Input: part model. Units: mm. Frame: model coordinates. A direction names the side the tool comes from. Coordinates: 2 decimals unless noted, no trailing zeros. Loops run counter-clockwise (first coordinate to the right, second up) from the corner with the lowest first, then second, coordinate; pieces in that order, holes last. Notation, with made-up numbers: (-35.5, -12) - (23.5, -12) arc R25 cw to (23.5, 15) - close; hole circle Ø4 at (-32, 5.25). An arc over 180 degrees is marked (long way). Use a Markdown table: item, result. Add a question column.
1. Access query for faces 1 (the face through (123.825, 47, 3)), 2 (the face through (93.967, 92, 3)), 3 (the face through (-82, 74.261, 3)). Directions: +Z, -Z, +X, -X, +Y, -Y. A direction counts if a zero-diameter tool reaches every point of the face in a straight line with its end or side. Return the directions, or none.
2. Ray query, L1, parallel to Y at x = 113, z = 2.5; L2, parallel to X at y = 88.5, z = 4.25; L3, parallel to X at y = 78, z = 5 (3 decimals). Return the intervals inside material, ascending. Write a range as [from, to].
3. Section query A-A on y = 14. Return the cut outline in (x, z).
4. Draft query along X for faces 4 (the face through (127, 38, 3)), 5 (the face through (62.23, 92, 3)), 6 (the face through (-19, 0, 3)). Return one class per face: released by +X, released by -X, zero draft, split by the parting line, or undercut.
5. Contact query for flat-ended pins moving along their axis: P1, Ø1.5, axis at y = 42.5, z = 4, coming from the -X side; P2, Ø3, axis at y = 25, z = 3.5, coming from the +X side (3 decimals); P3, Ø0.8, axis at x = 94.5, z = 2.5, coming from the -Y side. Output: stop coordinate, or through.
```python
from build123d import *

# Parameters (mm, degrees)
BOSS_EXTRUDE1_DEPTH     = 6.35
CUT_EXTRUDE4_DEPTH      = 127
CUT_EXTRUDE4_DEPTH_BACK = 127
CUT_EXTRUDE5_DEPTH      = 127
CUT_EXTRUDE5_DEPTH_BACK = 127
SKETCH5_W               = 229.808362084
SKETCH5_H               = 77.917038349
CUT_EXTRUDE7_DEPTH      = 127
CUT_EXTRUDE7_DEPTH_BACK = 127


with BuildPart() as part:
    # Sketch1 → Boss-Extrude1 (new body)
    with BuildSketch(Plane.XY):
        Polygon((0, 0), (127, 0), (127, 101.6), (0, 101.6), (-70.692427737, 172.292427737), (-91.896861793, 151.087993682), (-91.896861793, 0), align=None)
    extrude(amount=BOSS_EXTRUDE1_DEPTH)

    # Sketch3 → Cut-Extrude4 (cut, two sides)
    with BuildSketch(Plane(origin=(0, 0, 0), x_dir=(-1, 0, 0), z_dir=(0, 0, -1))) as cut_extrude4_sk:
        Polygon((-88.9, 101.6), (-101.6, 101.6), (-101.6, 98.425), (-96.5327, 98.425), (-96.5327, 85.725), (-93.9673, 85.725), (-93.9673, 98.425), (-88.9, 98.425), align=None)
        Polygon((-57.15, 101.6), (-69.85, 101.6), (-69.85, 98.425), (-64.77, 98.425), (-64.77, 85.725), (-62.23, 85.725), (-62.23, 98.425), (-57.15, 98.425), align=None)
        Polygon((-127, 82.55), (-127, 69.85), (-123.825, 69.85), (-123.825, 74.9173), (-111.125, 74.9173), (-111.125, 77.4827), (-123.825, 77.4827), (-123.825, 82.55), align=None)
        Polygon((-127, 57.15), (-127, 44.45), (-123.825, 44.45), (-123.825, 49.5173), (-111.125, 49.5173), (-111.125, 52.0827), (-123.825, 52.0827), (-123.825, 57.15), align=None)
        Polygon((-127, 31.75), (-127, 25.4), (-127, 19.05), (-123.825, 19.05), (-123.825, 24.1173), (-111.125, 24.1173), (-111.125, 26.6827), (-123.825, 26.6827), (-123.825, 31.75), align=None)
        Polygon((-101.6, 3.302), (-101.6, 0), (-88.9, 0), (-88.9, 3.302), (-93.9673, 3.302), (-93.9673, 16.002), (-96.5327, 16.002), (-96.5327, 3.302), align=None)
        Polygon((-25.4, 3.302), (-25.4, 0), (-12.7, 0), (-12.7, 3.302), (-17.7673, 3.302), (-17.7673, 16.002), (-20.3327, 16.002), (-20.3327, 3.302), align=None)
        Polygon((50.8, 3.302), (50.8, 0), (63.5, 0), (63.5, 3.302), (58.4327, 3.302), (58.4327, 16.002), (55.8673, 16.002), (55.8673, 3.302), align=None)
        Polygon((88.721861793, 31.42199842), (91.896861793, 31.42199842), (91.896861793, 44.12199842), (88.721861793, 44.12199842), (88.721861793, 39.05469842), (76.021861793, 39.05469842), (76.021861793, 36.48929842), (88.721861793, 36.48929842), align=None)
        Polygon((88.721861793, 69.193996841), (91.896861793, 69.193996841), (91.896861793, 81.893996841), (88.721861793, 81.893996841), (88.721861793, 76.826696841), (76.021861793, 76.826696841), (76.021861793, 74.261296841), (88.721861793, 74.261296841), align=None)
        Polygon((88.721861793, 106.965995261), (91.896861793, 106.965995261), (91.896861793, 119.665995261), (88.721861793, 119.665995261), (88.721861793, 114.598695261), (76.021861793, 114.598695261), (76.021861793, 112.033295261), (88.721861793, 112.033295261), align=None)
        Polygon((70.692427737, 158.822043556), (66.202299677, 154.331915495), (63.957235647, 156.576979525), (68.447363707, 161.067107586), align=None)
    extrude(amount=CUT_EXTRUDE4_DEPTH, mode=Mode.SUBTRACT)
    extrude(cut_extrude4_sk.sketch, amount=-CUT_EXTRUDE4_DEPTH_BACK, mode=Mode.SUBTRACT)

    # Sketch4 → Cut-Extrude5 (cut, two sides)
    with BuildSketch(Plane.XY) as cut_extrude5_sk:
        Polygon((-81.917747889, 147.596723404), (-79.672683858, 149.841787435), (-75.182555798, 145.351659374), (-77.427619828, 143.106595344), align=None)
    extrude(amount=CUT_EXTRUDE5_DEPTH, mode=Mode.SUBTRACT)
    extrude(cut_extrude5_sk.sketch, amount=-CUT_EXTRUDE5_DEPTH_BACK, mode=Mode.SUBTRACT)

    # Sketch5 → Cut-Extrude7 (cut, two sides)
    with BuildSketch(Plane.XY) as cut_extrude7_sk:
        with Locations((12.095818958, 140.558519175)):
            Rectangle(SKETCH5_W, SKETCH5_H)
    extrude(amount=CUT_EXTRUDE7_DEPTH, mode=Mode.SUBTRACT)
    extrude(cut_extrude7_sk.sketch, amount=-CUT_EXTRUDE7_DEPTH_BACK, mode=Mode.SUBTRACT)


solid = part.part
```
Resolved:
| question | item | result |
|---|---|---|
| 1 | face 1 | +Z, -Z, +X |
| 1 | face 2 | +Z, -Z, +Y |
| 1 | face 3 | +Z, -Z, -X |
| 2 | L1 | [0, 24.12], [26.68, 49.52], [52.08, 74.92], [77.48, 101.6] |
| 2 | L2 | [-91.9, 62.23], [64.77, 93.97], [96.53, 127] |
| 2 | L3 | [-88.722, 123.825] |
| 3 | outline | (-91.9, 0) - (-58.43, 0) - (-58.43, 6.35) - (-91.9, 6.35) - close; (-55.87, 0) - (17.77, 0) - (17.77, 6.35) - (-55.87, 6.35) - close; (20.33, 0) - (93.97, 0) - (93.97, 6.35) - (20.33, 6.35) - close; (96.53, 0) - (127, 0) - (127, 6.35) - (96.53, 6.35) - close |
| 4 | face 4 | released by +X |
| 4 | face 5 | undercut |
| 4 | face 6 | zero draft |
| 5 | P1 | x = -88.72 |
| 5 | P2 | x = 123.825 |
| 5 | P3 | y = 16 |
